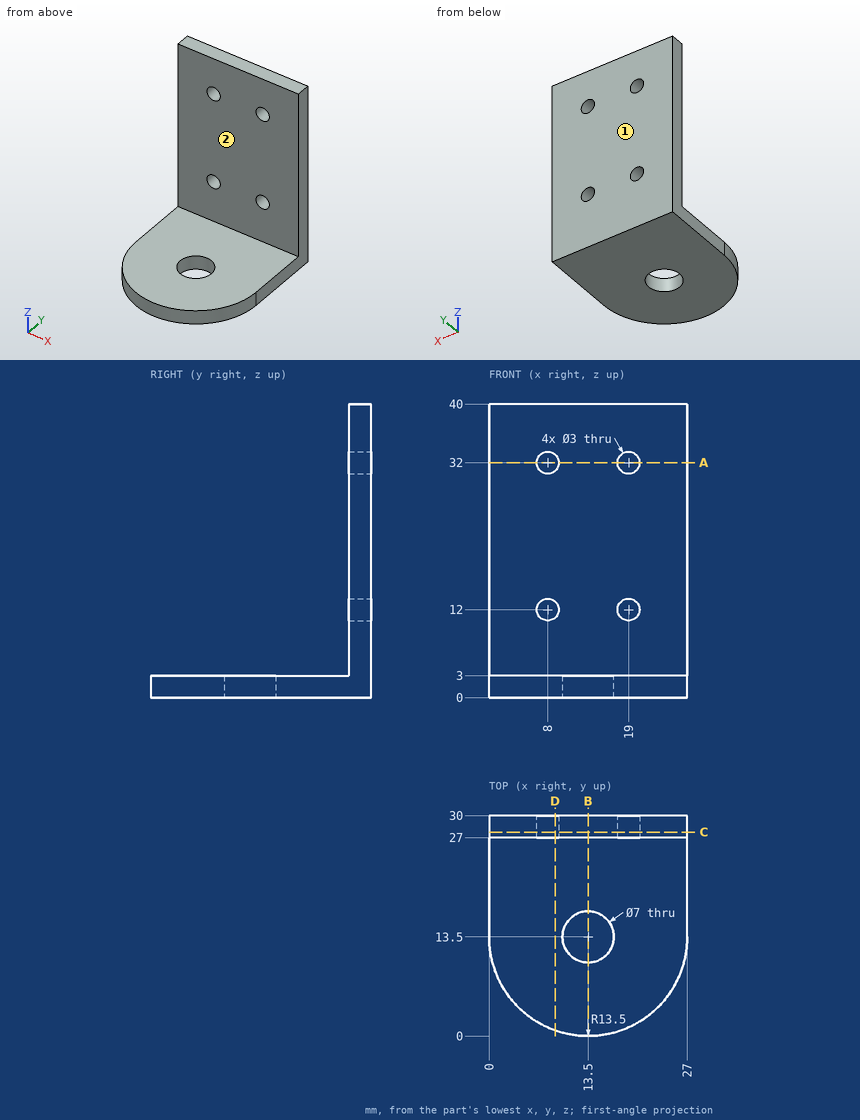
Design review of the part shown in the three views and the two pictorial views. Dimensions are in mm from the part's minimum x, y and z. A direction names the side the tool comes from. Give positions to 0.01 mm unless a question says otherwise; leave off trailing zeros. Write each loop counter-clockwise with the first axis right and the second up, starting at its lowest first coordinate (ties: lowest second). Pieces come first, ordered by that corner, then holes. Notation, with made-up numbers: M -7,-27.5 L 27,-27.5 A21 cw 27,1.5 Z; hole C 62.5,54.5 d5. An arc over 180 degrees is marked long. Return JSON: item names as keys, results as strings. Group by question number.
Item 1: Take a section at D-D (x = 9). Give the boundary of the cut face in (y, z).
Item 2: Clearance check with flat-ended pins moving along their axes: pin 1 Ø1.5 at (x, y) = (5, 17.5) entering from +Z; pin 2 Ø3.5 at (x, z) = (19, 12) entering from +Y; pin 3 Ø5 at (x, z) = (8, 32) entering from -Y; pin 4 Ø1.8 at (x, z) = (19, 32) entering from +Y. State where each tip first meets the part, or that it passes through.
Item 3: Wall thickness on line 1 along X through (y, z) = (28.2, 32); line 2 along Z through (x, y) = (19, 29.1); line 3 along X through (y, z) = (13.5, 0.65): over which ranges is each line inside the solid? List them lowest first.
Item 4: Take a section at C-C (y = 27.75). Give the boundary of the cut face in (x, z), plus the area to 3 significant figures.
Item 5: Tool access review of the marked faces 1 and 2: name each direction out of +Z, -Z, +X, -X, +Y, -Y from which nothing blocks a thin tool from reaching the whole face with its end or side.
Item 6: Take a section at B-B (x = 13.5). Give the boundary of the cut face in (y, z).
Item 7: Take a section at A-A (z = 32). Give the boundary of the cut face in (x, y), plus the area to 3 significant figures.
Return value:
{
 "1": {"outline": "M 0.77,0 L 30,0 L 30,10.88 L 27,10.88 L 27,3 L 0.77,3 Z; M 27,13.12 L 30,13.12 L 30,30.88 L 27,30.88 Z; M 27,33.12 L 30,33.12 L 30,40 L 27,40 Z"},
 "2": {"pin 1": "stops at z = 3", "pin 2": "stops at y = 30", "pin 3": "stops at y = 27", "pin 4": "passes through"},
 "3": {"line 1": "x = 0 to 6.5, 9.5 to 17.5, 20.5 to 27", "line 2": "z = 0 to 10.5, 13.5 to 30.5, 33.5 to 40", "line 3": "x = 0 to 10, 17 to 27"},
 "4": {"outline": "M 0,0 L 27,0 L 27,40 L 0,40 Z; hole C 8,12 d3; hole C 8,32 d3; hole C 19,12 d3; hole C 19,32 d3", "area": "1,050 mm2"},
 "5": {"face 1": "+Z, -Z, +X, -X, +Y", "face 2": "+Z, +X, -X, -Y"},
 "6": {"outline": "M 0,0 L 10,0 L 10,3 L 0,3 Z; M 17,0 L 30,0 L 30,40 L 27,40 L 27,3 L 17,3 Z"},
 "7": {"outline": "M 0,27 L 6.5,27 L 6.5,30 L 0,30 Z; M 9.5,27 L 17.5,27 L 17.5,30 L 9.5,30 Z; M 20.5,27 L 27,27 L 27,30 L 20.5,30 Z", "area": "63.0 mm2"}
}
